Source: CAD feature listing. Evaluate the final solid. Frame: model axes, mm. A direction names the side the tool comes from. Coordinates: 2 decimals unless noted, no trailing zeros. Order: outer loops, then holes, each group sorted by start corner. A loop starts at its lowest first (then second) coordinate and runs counter-clockwise, first axis right, second up.
Item 1: Section D-D on z = 12.5. Return the cut outline in (x, y), then the cut area to 3 significant figures.
Item 2: Section B-B on x = -2.25. Return the cut outline in (y, z) (3 decimals), then the cut area to 3 significant figures.
Item 3: Section C-C on y = 0. State how many separate pieces and enclosed holes the cut face has, then the cut area to 3 significant figures.
Item 4: Reachability of faces 1 (the flat face through (0, 3, -11)), 2 (the flat face through (-0.255, -3, -10)), 3 (the cylindrical face through (-9.661, 5.774, 1.282)) from +Z, -Z, +X, -X, +Y, -Y: full face, straight path, thin tool, end or side. Return the list, or none.
Item 5: Mould query, pull axis Z, two halves, no side actions, for faces 4 (the cylindrical face through (-2, 0, 24)), 5 (the cylindrical face through (-1.972, 0.115, -15.378)), 6 (the flat face through (-8.4, 10, -6)). Classes: released by +Z, released by -Z, zero draft, split by the parting line, or undercut.
Item 6: Ray query, line 1 (Y direction, x = -8.1, z = 0) (3 decimals); line 2 (X direction, y = 2.75, z = 5.5). Return the intervals inside material, ascending.
Item 7: Contact query for flat-ended pins moving along their axis: P1, Ø13, axis at y = 0, z = 0, coming from the -X side; P2, Ø4, axis at x = -6.5, y = -8, coming from the +Z side; P3, Ø2, axis at x = -5.5, z = 12.5, coming from the +Y side; P4, Ø2, axis at y = 6.5, z = 18, coming from the -X side. Output: stop coordinate, or through.
from build123d import *

# Parameters (mm, degrees)
SKETCH4_R           = 11.2
SKETCH4_R_2         = 2.625
BOSS_EXTRUDE3_DEPTH = 4


with BuildPart() as part:
    # Sketch2 → Revolve1 (revolve)
    with BuildSketch(Plane(origin=(0, 0, 0), x_dir=(1, 0, 0), z_dir=(0, 1, 0))):
        Polygon((-0.255431619, 4), (-11.7, 4), (-11.7, 5.915), (-7.678354549, 5.915), (-7.678354549, 10.2), (-7.915390692, 10.2), (-7.915390692, 11.2), (-8.1271402, 11.2), (-8.4, 11.4728598), (-8.4, 13.5), (0, 13.5), (0, 11.2), (-0.255431619, 11.2), (-0.255431619, 10.2), (-0.384561477, 10.2), (-0.384561477, 5.915), (-0.255431619, 5.915), align=None)
    revolve(axis=Axis((0, 0, 0), (-1, 0, 0)))

    # Sketch4 → Boss-Extrude3 (add)
    with BuildSketch(Plane(origin=(0, 0, 0), x_dir=(0, 0, -1), z_dir=(1, 0, 0))):
        with BuildLine():
            ThreePointArc((20.5, 5.454356057), (24, 0), (20.5, -5.454356057))
            Line((20.5, -5.454356057), (5.625, -12.272301129))
            ThreePointArc((5.625, -12.272301129), (0, -13.5), (-5.625, -12.272301129))
            Line((-5.625, -12.272301129), (-20.5, -5.454356057))
            ThreePointArc((-20.5, -5.454356057), (-24, 0), (-20.5, 5.454356057))
            Line((-20.5, 5.454356057), (-5.625, 12.272301129))
            ThreePointArc((-5.625, 12.272301129), (0, 13.5), (5.625, 12.272301129))
            Line((5.625, 12.272301129), (20.5, 5.454356057))
        make_face()
        Circle(SKETCH4_R, mode=Mode.SUBTRACT)
        with Locations((-18, 0)):
            Circle(SKETCH4_R_2, mode=Mode.SUBTRACT)
        with Locations((18, 0)):
            Circle(SKETCH4_R_2, mode=Mode.SUBTRACT)
    extrude(amount=-BOSS_EXTRUDE3_DEPTH)


solid = part.part
Answer list:
1. outline: (-8.4, -5.1) - (-4, -5.1) - (-4, -9.12) - (0, -9.12) - (0, 9.12) - (-4, 9.12) - (-4, 5.1) - (-8.4, 5.1) - close
1. area: 118 mm2
2. outline: (-12.272, -5.625) - (-5.454, -20.5) arc R6 ccw to (5.454, -20.5) - (12.272, -5.625) arc R13.5 ccw to (12.272, 5.625) - (5.454, 20.5) arc R6 ccw to (-5.454, 20.5) - (-12.272, 5.625) arc R13.5 ccw to start; hole circle Ø8 at (0, 0); hole circle Ø5.25 at (0, -18); hole circle Ø5.25 at (0, 18)
2. area: 783 mm2
3. separate pieces: 4
3. enclosed holes: 0
3. area: 202 mm2
4. face 1: +Z, -Z, +X, +Y, -Y
4. face 2: +X
4. face 3: -X
5. face 4: released by +Z
5. face 5: undercut
5. face 6: zero draft
6. line 1: y = -13.5 to -11.2, -5.915 to -4, 4 to 5.915, 11.2 to 13.5
6. line 2: x = -7.68 to -0.38
7. P1: stops at x = -11.7
7. P2: stops at z = 12.09
7. P3: stops at y = 7.07
7. P4: stops at x = -4
